```python
from build123d import *

# Parameters (mm, degrees)
F0_R     = 9.525
F1_DEPTH = 25.4
F3_DEPTH = 25.401
F4_DEPTH = 11.1125
F6_DEPTH = 9.525


with BuildPart() as f1:
    # F0 (on Front) → F1 (new body)
    with BuildSketch(Plane.XZ):
        Circle(F0_R)
    extrude(amount=-F1_DEPTH)

    # F2 (on face) → F3 (cut, through all)
    with BuildSketch(Plane(origin=(0, 25.4, 0), x_dir=(-1, 0, 0), z_dir=(0, 1, 0))):
        with BuildLine():
            ThreePointArc((-4.7625, 0), (-3.367596, -3.367596), (0, -4.7625))
            ThreePointArc((0, -4.7625), (3.367596, -3.367596), (4.7625, 0))
            ThreePointArc((4.7625, 0), (3.367596, 3.367596), (0, 4.7625))
            ThreePointArc((0, 4.7625), (-3.367596, 3.367596), (-4.7625, 0))
        make_face()
    extrude(amount=-F3_DEPTH, mode=Mode.SUBTRACT)

    # F2 (on face) → F4 (cut)
    with BuildSketch(Plane(origin=(0, 25.4, 0), x_dir=(-1, 0, 0), z_dir=(0, 1, 0))):
        with BuildLine():
            Line((-4.7625, 0), (-4.7625, -4.7625))
            Line((-4.7625, -4.7625), (0, -4.7625))
            ThreePointArc((0, -4.7625), (-3.367596, -3.367596), (-4.7625, 0))
        make_face()
        with BuildLine():
            ThreePointArc((4.7625, 0), (3.367596, -3.367596), (0, -4.7625))
            Line((0, -4.7625), (4.7625, -4.7625))
            Line((4.7625, -4.7625), (4.7625, 0))
        make_face()
        with BuildLine():
            Line((-4.7625, 4.7625), (-4.7625, 0))
            ThreePointArc((-4.7625, 0), (-3.367596, 3.367596), (0, 4.7625))
            Line((0, 4.7625), (-4.7625, 4.7625))
        make_face()
        with BuildLine():
            ThreePointArc((0, 4.7625), (3.367596, 3.367596), (4.7625, 0))
            Line((4.7625, 0), (4.7625, 4.7625))
            Line((4.7625, 4.7625), (0, 4.7625))
        make_face()
    extrude(amount=-F4_DEPTH, mode=Mode.SUBTRACT)

    # F5 (on face) → F6 (cut)
    with BuildSketch(Plane.XZ):
        Polygon((-7.332348, 0), (-3.666174, -6.35), (3.666174, -6.35), (7.332348, 0), (3.666174, 6.35), (-3.666174, 6.35), align=None)
    extrude(amount=-F6_DEPTH, mode=Mode.SUBTRACT)


solid = f1.part
```
Input: part model. Units: mm. Frame: model coordinates. A direction names the side the tool comes from. Round coordinates to 2 decimals unless told otherwise and drop trailing zeros. Loops run counter-clockwise (first coordinate to the right, second up) from the corner with the lowest first, then second, coordinate; pieces in that order, holes last.
1) Section query C-C on z = 3. Return the cut outline in (x, y) (1 decimal), plus the area to 3 significant figures.
Ans:
outline: (-9, 0) - (-5.6, 0) - (-5.6, 9.5) - (-3.7, 9.5) - (-3.7, 14.3) - (-4.8, 14.3) - (-4.8, 25.4) - (-9, 25.4) - close; (3.7, 9.5) - (5.6, 9.5) - (5.6, 0) - (9, 0) - (9, 25.4) - (4.8, 25.4) - (4.8, 14.3) - (3.7, 14.3) - close
area: 211 mm2
2) Material intervals for line 1 (Z direction, x = -6.25, y = 7.5); line 2 (Z direction, x = 6, y = 4); line 3 (Z direction, x = 8.25, y = 9.25), sorted ascending.
Ans:
line 1: z = -7.19 to -1.87, 1.87 to 7.19
line 2: z = -7.4 to -2.31, 2.31 to 7.4
line 3: z = -4.76 to 4.76
3) Pin query (flat end, axial travel): pin 1 (10.5 mm diameter, centred on x = 2, y = 17.5, fed in from +Z) (3 decimals); pin 2 (2 mm diameter, centred on y = 16, z = 5, fed in from -X); pin 3 (6 mm diameter, centred on x = 7, y = 6.5, fed in from +Z); pin 4 (2 mm diameter, centred on y = 12.5, z = 3.5, fed in from -X). Return the tip coordinate at first contact, or that it passes through.
Ans:
pin 1: stops at z = 9.525
pin 2: stops at x = -8.64
pin 3: stops at z = 8.64
pin 4: stops at x = -9.19
4) Pull-direction query (Z, two-part tool) for faces 1 (the cylindrical face through (-7.559, 12.522, -5.796)), 2 (the flat face through (-5.525, 4.696, -3.131)), 3 (the flat face through (6.2, 0, 2.3)); classes: released by +Z, released by -Z, zero draft, split by the parting line, or undercut.
Ans:
face 1: split by the parting line
face 2: undercut
face 3: zero draft
5) Section query A-A on y = 4.25. Return the cut outline in (x, z) (3 decimals).
Ans:
outline: circle Ø19.05 at (0, 0); hole (-7.332, 0) - (-3.666, -6.35) - (3.666, -6.35) - (7.332, 0) - (3.666, 6.35) - (-3.666, 6.35) - close
6) Set-up query: faces 4 (the flat face through (0, 25.4, -6)), 5 (the flat face through (-4.762, 20, 0)), 6 (the flat face through (5.474, 4.696, -3.219)). Return all of +Z, -Z, +X, -X, +Y, -Y with unobstructed straight access to the full face (end or side cutting, diameter ignored); none if empty.
Ans:
face 4: +Z, -Z, +X, -X, +Y
face 5: +Y
face 6: -Y
